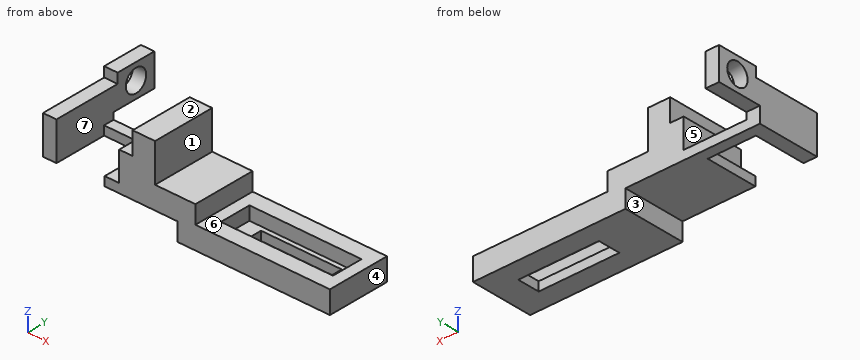
from build123d import *

# Parameters (mm, degrees)
BOSS_EXTRUDE1_DEPTH      = 14
SKETCH2_W                = 25
SKETCH2_H                = 7
CUT_EXTRUDE3_DEPTH       = 3
SKETCH10_W               = 18
SKETCH10_H               = 5
CUT_EXTRUDE4_DEPTH       = 68.321987493
BOSS_EXTRUDE8_DEPTH      = 3
SKETCH15_R               = 2.5
CUT_EXTRUDE8_DEPTH       = 71.556714776
CUT_EXTRUDE11_DEPTH      = 7
CUT_EXTRUDE11_DEPTH_BACK = 7
SKETCH18_W               = 6.5
SKETCH18_H               = 14
SKETCH19_W               = 10.762656819
SKETCH19_H               = 11.671990231
CUT_EXTRUDE12_DEPTH      = 7


with BuildPart() as part:
    # Sketch1 → Boss-Extrude1 (new body)
    with BuildSketch(Plane(origin=(0, 0, 0), x_dir=(1, 0, 0), z_dir=(0, 1, 0))):
        Polygon((25, 0), (25, 8.5), (34, 8.5), (34, 12.5), (64, 12.5), (64, 17.5), (30, 17.5), (30, 13.5), (0, 13.5), (0, 5), (20, 5), (20, 0), align=None)
    extrude(amount=BOSS_EXTRUDE1_DEPTH)

    # Sketch2 → Cut-Extrude3 (cut)
    with BuildSketch(Plane.XY.offset(-12.5)):
        with Locations((49, 7)):
            Rectangle(SKETCH2_W, SKETCH2_H)
    extrude(amount=-CUT_EXTRUDE3_DEPTH, mode=Mode.SUBTRACT)

    # Sketch10 → Cut-Extrude4 (cut, through all)
    with BuildSketch(Plane.XY.offset(-15.5)):
        with Locations((49, 7)):
            Rectangle(SKETCH10_W, SKETCH10_H)
    extrude(amount=-CUT_EXTRUDE4_DEPTH, mode=Mode.SUBTRACT)

    # Sketch11 → Boss-Extrude8 (add)
    with BuildSketch(Plane.ZY):
        Polygon((-10, 14), (-10, 24), (-2.800888244, 24), (-2.800888244, 15), (-5, 15), (-5, 14), align=None)
    extrude(amount=-BOSS_EXTRUDE8_DEPTH)

    # Sketch15 → Cut-Extrude8 (cut, through all)
    with BuildSketch(Plane.ZY):
        with Locations((-6.400444122, 19.5)):
            Circle(SKETCH15_R)
    extrude(amount=-CUT_EXTRUDE8_DEPTH, mode=Mode.SUBTRACT)

    # Sketch18 → Cut-Extrude11 (cut, two sides: drawn at the far end of the back side and taken through both)
    with BuildSketch(Plane.ZY.offset(-10).offset(-CUT_EXTRUDE11_DEPTH_BACK)):
        with Locations((-8.25, 7)):
            Rectangle(SKETCH18_W, SKETCH18_H)
    extrude(amount=CUT_EXTRUDE11_DEPTH + CUT_EXTRUDE11_DEPTH_BACK, mode=Mode.SUBTRACT)

    # Sketch19 → Cut-Extrude12 (cut)
    with BuildSketch(Plane(origin=(0, 0, -13.5), x_dir=(-1, 0, 0), z_dir=(0, 0, -1))):
        with Locations((-8.38132841, 5.835995116)):
            Rectangle(SKETCH19_W, SKETCH19_H)
    extrude(amount=-CUT_EXTRUDE12_DEPTH, mode=Mode.SUBTRACT)


solid = part.part
Work out the finished part from the listing and answer in its coordinate system (mm). Face numbers are marked on the shaded views. A direction names the side the tool comes from. Round coordinates to 2 decimals unless told otherwise and drop trailing zeros. Write each loop counter-clockwise with the first axis right and the second up, starting at its lowest first coordinate (ties: lowest second). Pieces come first, ordered by that corner, then holes.
1) A tool of negligible diameter and unlimited length cuts with its end or side. For the marked faces 1, 2 and 3, from which of +Z, -Z, +X, -X, +Y, -Y can it reach the whole face along a straight path? Write none if from no direction.
2) A cutting plane is placed at D-D (x = 60). Give the vertices of the cut face in (y, z).
3) A cutting plane is placed at A-A (y = 7). Give the vertices of the cut face in (x, z).
4) Given pin 1 Ø10 at (y, z) = (15, -5.5) entering from +X; pin 2 Ø8 at (x, y) = (30.5, 17.5) entering from +Z; pin 3 Ø1.5 at (x, z) = (31, -15.5) entering from +Y; pin 4 Ø4 at (x, y) = (10.5, 7.5) entering from +Z, each flat-ended and moving along its own axis, determine where each tip first touches the part or whether it passes through.
5) The mould has two halves that part along X. Classify the marked faces 4, 5, 6 and 7: pulls with the +X half, pulls with the -X half, needs draft (parallel to the pull), parting line crosses it, or undercut.
6) Straight lines are drawn through the part: line 1 (X direction, y = 11, z = -10.5); line 2 (X direction, y = 3.5, z = -6.5); line 3 (Y direction, x = 16, z = -11.75). For each, find the intervals that lie inside material, in ascending order.
7) A cutting plane is placed at C-C (y = 19.5). Give the vertices of the cut face in (x, z).
8) A cutting plane is placed at B-B (x = 45). Give the vertices of the cut face in (y, z).
Completed:
1. face 1: +Z, +X, +Y, -Y
1. face 2: +Z, +X, -X, +Y, -Y
1. face 3: -Z, -X, +Y, -Y
2. outline: (0, -17.5) - (14, -17.5) - (14, -12.5) - (10.5, -12.5) - (10.5, -15.5) - (3.5, -15.5) - (3.5, -12.5) - (0, -12.5) - close
3. outline: (0, -13.5) - (3, -13.5) - (3, -5) - (0, -5) - close; (13.76, -13.5) - (30, -13.5) - (30, -17.5) - (40, -17.5) - (40, -15.5) - (36.5, -15.5) - (36.5, -12.5) - (34, -12.5) - (34, -8.5) - (25, -8.5) - (25, 0) - (20, 0) - (20, -5) - (17, -5) - (17, -11.5) - (13.76, -11.5) - close; (58, -17.5) - (64, -17.5) - (64, -12.5) - (61.5, -12.5) - (61.5, -15.5) - (58, -15.5) - close
4. pin 1: stops at x = 34
4. pin 2: stops at z = -8.5
4. pin 3: stops at y = 14
4. pin 4: passes through
5. face 4: pulls with the +X half
5. face 5: undercut
5. face 6: needs draft
5. face 7: undercut
6. line 1: x = 0 to 3, 17 to 34
6. line 2: x = 0 to 3, 17 to 25
6. line 3: y = 0 to 14
7. outline: (0, -10) - (3, -10) - (3, -8.9) - (0, -8.9) - close; (0, -3.9) - (3, -3.9) - (3, -2.8) - (0, -2.8) - close
8. outline: (0, -17.5) - (4.5, -17.5) - (4.5, -15.5) - (3.5, -15.5) - (3.5, -12.5) - (0, -12.5) - close; (9.5, -17.5) - (14, -17.5) - (14, -12.5) - (10.5, -12.5) - (10.5, -15.5) - (9.5, -15.5) - close
